```python
from build123d import *

# Parameters (mm, degrees)
F1_DEPTH  = 182.5
F3_DEPTH  = 200
F5_DEPTH  = 200
F7_DEPTH  = 220.001
F8_W      = 138
F8_H      = 20
F8_H_2    = 24
F9_DEPTH  = 365.001
F12_DEPTH = 35
F10_R     = 3.4
F14_DEPTH = 22.3866406461
F13_R     = 3.4
F15_DEPTH = 25
F16_DEPTH = 25


with BuildPart() as f1:
    # F0 (on Front) → F1 (new body, symmetric)
    with BuildSketch(Plane.XZ):
        Polygon((110, 0), (-110, 0), (-110, -33), (-86, -38), (-86, -110), (92, -110), (92, -38), (110, -33), align=None)
    extrude(amount=F1_DEPTH, both=True)

    # F2 (on Front) → F3 (cut, symmetric)
    with BuildSketch(Plane.XZ):
        Polygon((84.9585481157, 0), (-80.3397459622, 0), (-89.5773502692, -16), (94.1961524227, -16), align=None)
    extrude(amount=F3_DEPTH, both=True, mode=Mode.SUBTRACT)

    # F4 (on Right) → F5 (cut, symmetric)
    with BuildSketch(Plane.YZ):
        Polygon((-74.5, -90), (-74.5, -110), (56.9529946162, -110), (68.5, -90), align=None)
    extrude(amount=F5_DEPTH, both=True, mode=Mode.SUBTRACT)

    # F6 (on face) → F7 (cut, through all)
    with BuildSketch(Plane.YZ.offset(110)):
        Polygon((-102.5, -80), (-182.5, -40), (-182.5, -150), (-92.5, -150), (-92.5, -80), align=None)
        Polygon((182.5, -150), (182.5, -40), (102.5, -80), (92.5, -80), (92.5, -150), align=None)
    extrude(amount=-F7_DEPTH, mode=Mode.SUBTRACT)

    # F8 (on face) → F9 (cut, through all)
    with BuildSketch(Plane.XZ.offset(182.5)):
        with Locations((3, -50)):
            Rectangle(F8_W, F8_H)
        with Locations((3, -28)):
            Rectangle(F8_W, F8_H_2)
    extrude(amount=-F9_DEPTH, mode=Mode.SUBTRACT)

    # F11 (on face) → F12 (cut)
    with BuildSketch(Plane.YZ.offset(110)):
        with BuildLine():
            Line((-3.9452221542, -33), (4.9452221542, -33))
            ThreePointArc((4.9452221542, -33), (0.5, -30.4), (-3.9452221542, -33))
        make_face()
        with BuildLine():
            ThreePointArc((-3.9452221542, -33), (-0.7921623377, -40.4335906289), (5.6, -35.5))
            ThreePointArc((5.6, -35.5), (5.4335906289, -34.2078376623), (4.9452221542, -33))
            Line((4.9452221542, -33), (-3.9452221542, -33))
        make_face()
    extrude(amount=-F12_DEPTH, mode=Mode.SUBTRACT)

    # F10 (on face) → F14 (cut, through all)
    with BuildSketch(Plane.YZ.offset(110)):
        with Locations((-165, -8)):
            Circle(F10_R)
        with Locations((-86.5, -8)):
            Circle(F10_R)
        with Locations((-7.5, -8)):
            Circle(F10_R)
        with Locations((74, -8)):
            Circle(F10_R)
        with Locations((154, -8)):
            Circle(F10_R)
    extrude(amount=-F14_DEPTH, mode=Mode.SUBTRACT)

    # F13 (on face) → F15 (cut)
    with BuildSketch(Plane.YZ.offset(110)):
        with Locations((-59.5, -23)):
            Circle(F13_R)
        with Locations((60.5, -23)):
            Circle(F13_R)
    extrude(amount=-F15_DEPTH, mode=Mode.SUBTRACT)

    # F13 (on face) → F16 (cut)
    with BuildSketch(Plane.YZ.offset(110)):
        with Locations((-59.5, -23)):
            Circle(F13_R)
        with Locations((60.5, -23)):
            Circle(F13_R)
    extrude(amount=-F16_DEPTH, mode=Mode.SUBTRACT)


solid = f1.part
```
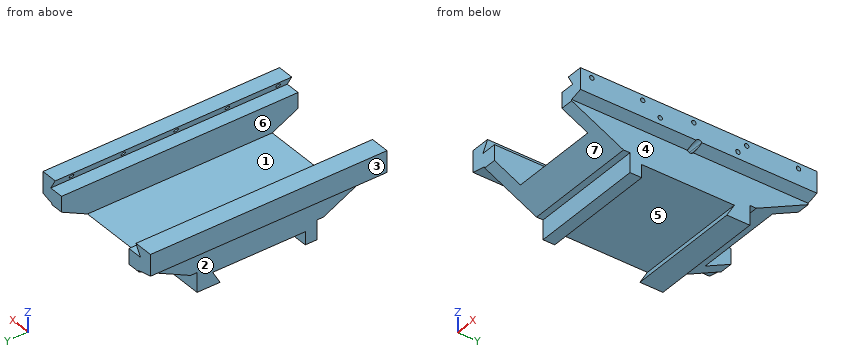
Source: CAD feature listing. Evaluate the final solid. Frame: model axes, mm. Face numbers are marked on the shaded views. A direction names the side the tool comes from. Coordinates: 2 decimals unless noted, no trailing zeros. Order: outer loops, then holes, each group sorted by start corner. A loop starts at its lowest first (then second) coordinate and runs counter-clockwise, first axis right, second up. Notation, with made-up numbers: M 53.25,67.5 L 75.25,67.5 A26 ccw 75.25,92.5 Z; hole C 88.25,3.5 d3. An arc over 180 degrees is marked long. Write each question's results on one line, items separated by ' | '. Start each with the question number.
1) Contact query for flat-ended pins moving along their axis: pin 1 Ø2 at (x, z) = (20, -90.5) entering from -Y; pin 2 Ø5.5 at (y, z) = (74, -8) entering from +X; pin 3 Ø8 at (y, z) = (2, -67.5) entering from -X. Output: stop coordinate, or through.
2) Access query for the marked faces 1, 2, 3 and 4. Directions: +Z, -Z, +X, -X, +Y, -Y. A direction counts if a zero-diameter tool reaches every point of the face in a straight line with its end or side. Return the directions, or none.
3) Section query C-C (y = 0.5). Return the cut outline in (x, z), plus the area to 3 significant figures.
4) Section query B-B (z = -75.5). Return the cut outline in (x, y).
5) Section query A-A (y = -51). Return the cut outline in (x, z).
6) Line query: line 1 (Y direction, x = 98.5, z = -8); line 2 (X direction, y = 135, z = -32.5); line 3 (Y direction, x = 90, z = -35.5). Output: solid intervals per line, ascending. Write a range as from..to.
7) Draft query along Y for the marked faces 5, 6 and 7. Return one class per face: released by +Y, released by -Y, zero draft, split by the parting line, or undercut.
Answers:
1) pin 1: stops at y = -92.5 | pin 2: stops at x = -83.37 | pin 3: stops at x = -86
2) face 1: +Z, +Y, -Y | face 2: -Z, -X, +Y, -Y | face 3: +Z, -Z, -X, +Y, -Y | face 4: -Z, +X, +Y, -Y
3) outline: M -110,-33 L -86,-38 L -86,-90 L 92,-90 L 92,-40.6 L 75,-40.6 L 75,-30.4 L 110,-30.4 L 110,0 L 84.96,0 L 94.2,-16 L 72,-16 L 72,-60 L -66,-60 L -66,-16 L -89.58,-16 L -80.34,0 L -110,0 Z | area: 8,380 mm^2
4) outline: M -86,-111.5 L 92,-111.5 L 92,111.5 L -86,111.5 Z
5) outline: M -110,-33 L -86,-38 L -86,-90 L 92,-90 L 92,-38 L 110,-33 L 110,0 L 84.96,0 L 94.2,-16 L 72,-16 L 72,-60 L -66,-60 L -66,-16 L -89.58,-16 L -80.34,0 L -110,0 Z
6) line 1: y = -182.5..-168.4, -161.6..-89.9, -83.1..-10.9, -4.1..70.6, 77.4..150.6, 157.4..182.5 | line 2: x = -110..-66, 72..110 | line 3: y = -182.5..-4.6, 5.6..182.5
7) face 5: undercut | face 6: zero draft | face 7: released by -Y
